Could you check a few things on this model? Use its own coordinates, in mm. A direction names the side the tool comes from. Give positions to 0.01 mm unless a question says otherwise; leave off trailing zeros. Write each loop counter-clockwise with the first axis right and the second up, starting at its lowest first coordinate (ties: lowest second). Pieces come first, ordered by that corner, then holes. Notation, with made-up numbers: (49.25, -27) - (61.25, -27) arc R26 ccw to (61.25, 12) - close; hole circle Ø2 at (39.25, 51.5). An arc over 180 degrees is marked (long way). Write item = value, one per line.
from build123d import *

# Parameters (mm, degrees)
SKETCH1_R                       = 2.5
BOSS_EXTRUDE1_DEPTH             = 25
SKETCH9_W                       = 45.48
SKETCH9_H                       = 45
BOSS_EXTRUDE4_DEPTH             = 15
CUT_EXTRUDE2_START              = -2.5
CUT_EXTRUDE2_DEPTH              = 19.5
SKETCH15_R                      = 2.5
BOSS_EXTRUDE5_DEPTH             = 25
CHAMFER1_SIZE                   = 10
CUT_EXTRUDE3_REACH              = 47.48
SKETCH16_W                      = 40
SKETCH16_H                      = 19.5
SKETCH17_W                      = 15.08
SKETCH17_H                      = 6
BOSS_EXTRUDE6_DEPTH             = 22
CBORE_FOR_M5_SBHCS1_D           = 5.5
CBORE_FOR_M5_SBHCS1_CBORE_D     = 10.5
CBORE_FOR_M5_SBHCS1_CBORE_DEPTH = 9.75
CHAMFER2_SIZE                   = 0.5


with BuildPart() as part:
    # Sketch1 → Boss-Extrude1 (new body)
    with BuildSketch(Plane(origin=(0, 0, 0), x_dir=(1, 0, 0), z_dir=(0, 1, 0))):
        Polygon((20.24, -10), (25.24, -10), (25.24, 10), (20.24, 10), (-20.24, 10), (-20.24, -10), align=None)
        Circle(SKETCH1_R, mode=Mode.SUBTRACT)
    extrude(amount=BOSS_EXTRUDE1_DEPTH)

    # Sketch9 → Boss-Extrude4 (add)
    with BuildSketch(Plane.XY.offset(10)):
        with Locations((2.5, 2.5)):
            Rectangle(SKETCH9_W, SKETCH9_H)
    extrude(amount=BOSS_EXTRUDE4_DEPTH)

    # Sketch10 → Cut-Extrude2 (cut)
    with BuildSketch(Plane(origin=(0, 25, 0), x_dir=(1, 0, 0), z_dir=(0, 1, 0)).offset(CUT_EXTRUDE2_START)):
        with BuildLine():
            Line((10.16, 0), (10.16, 10))
            Line((10.16, 10), (-10.16, 10))
            Line((-10.16, 10), (-10.16, 0))
            ThreePointArc((-10.16, 0), (0, -10.16), (10.16, 0))
        make_face()
    extrude(amount=-CUT_EXTRUDE2_DEPTH, mode=Mode.SUBTRACT)

    # Sketch15 → Boss-Extrude5 (add)
    with BuildSketch(Plane(origin=(0, 25, 0), x_dir=(1, 0, 0), z_dir=(0, 1, 0))):
        with BuildLine():
            Line((25.24, 10), (25.24, 12.732395665))
            ThreePointArc((25.24, 12.732395665), (12.732395665, 25.24), (0.224791329, 12.732395665))
            Line((0.224791329, 12.732395665), (0.224791329, 10))
            Line((0.224791329, 10), (25.24, 10))
        make_face()
        with Locations((12.732395665, 12.732395665)):
            Circle(SKETCH15_R, mode=Mode.SUBTRACT)
    extrude(amount=-BOSS_EXTRUDE5_DEPTH)

    # Chamfer1
    chamfer1_edges = [part.edges().sort_by_distance(p)[0] for p in [
        (2.5, 25, 25),
    ]]
    chamfer(chamfer1_edges, length=CHAMFER1_SIZE)

    # Sketch16 → Cut-Extrude3 (cut, up to next)
    with BuildSketch(Plane(origin=(25.24, 0, 0), x_dir=(0, 0, -1), z_dir=(1, 0, 0)), mode=Mode.PRIVATE) as cut_extrude3_sk1:
        with Locations((9.84, 12.75)):
            Rectangle(SKETCH16_W, SKETCH16_H)
    cut_extrude3_tool1 = extrude(cut_extrude3_sk1.sketch, amount=-CUT_EXTRUDE3_REACH, mode=Mode.PRIVATE) & part.part
    add(cut_extrude3_tool1.solids().sort_by_distance((25.24, 12.75, -9.84))[0], mode=Mode.SUBTRACT)

    # Sketch17 → Boss-Extrude6 (add)
    with BuildSketch(Plane(origin=(0, 25, 0), x_dir=(1, 0, 0), z_dir=(0, 1, 0))):
        with Locations((17.7, 0)):
            Rectangle(SKETCH17_W, SKETCH17_H)
    extrude(amount=-BOSS_EXTRUDE6_DEPTH)

    # CBORE for M5 SBHCS1 (through all)
    with Locations(Plane.XY.offset(25)):
        with Locations((-13.24, -10), (18.24, -10)):
            CounterBoreHole(CBORE_FOR_M5_SBHCS1_D / 2, CBORE_FOR_M5_SBHCS1_CBORE_D / 2, CBORE_FOR_M5_SBHCS1_CBORE_DEPTH)

    # Chamfer2
    chamfer2_edges = [part.edges().sort_by_distance(p)[0] for p in [
        (-20.24, 25, 2.5),
        (-20.24, -20, 17.5),
        (25.24, -20, 17.5),
        (2.5, -20, 25),
        (25.24, -2.5, 25),
        (-10.007604335, 25, -10),
        (12.732395665, 25, -25.24),
        (0.224791329, 25, -11.366197832),
        (-20.24, -2.5, 25),
        (-20.24, 20, 20),
        (25.24, 25, 1.133802168),
        (25.24, 20, 20),
    ]]
    chamfer(chamfer2_edges, length=CHAMFER2_SIZE)


solid = part.part
1. Which directions (+Z, -Z, +X, -X, +Y, -Y) give clear straight access to the entire face, cutting with the end or side of a thin tool? Please do faces 4 (the face through (18, 13, 3)), 5 (the face through (-11, -12, 15.25)), 6 (the face through (-10.16, 13, -5)), 7 (the face through (25.24, 2.8, 10.3)), 8 (the face through (-15.78, -11.05, 12.59)).
Filled sheet:
face_4 = +X
face_5 = +Z
face_6 = -Z
face_7 = +Z, -Z, +X, +Y, -Y
face_8 = +Z, -Z
2. For pin 1 (0.6 mm diameter, centred on y = 23, z = -11, fed in from -X); pin 2 (2 mm diameter, centred on x = 18.5, y = 14, fed in from -Z); pin 3 (6 mm diameter, centred on x = -10.5, y = 12.5, fed in from -Z), each with a flat end and sliding along its axis, tell me the tip position at first contact or that it passes through.
Filled sheet:
pin_1 = 0.22
pin_2 = -3
pin_3 = -10
3. If we section it at C-C, the plane z = -7.5: Please give me the cut outline in (x, y).
Filled sheet:
outline = (-20.24, 0) - (25.24, 0) - (25.24, 3) - (-10.16, 3) - (-10.16, 22.5) - (25.24, 22.5) - (25.24, 24.5) - (24.74, 25) - (-19.74, 25) - (-20.24, 24.5) - close
4. If we section it at B-B, the plane y = -10: Please give me the cut outline in (x, z).
Filled sheet:
outline = (-20.24, 10) - (-15.99, 10) - (-15.99, 15.25) - (-18.49, 15.25) - (-18.49, 25) - (-19.74, 25) - (-20.24, 24.5) - close; (-10.49, 10) - (15.49, 10) - (15.49, 15.25) - (12.99, 15.25) - (12.99, 25) - (-7.99, 25) - (-7.99, 15.25) - (-10.49, 15.25) - close; (20.99, 10) - (25.24, 10) - (25.24, 24.5) - (24.74, 25) - (23.49, 25) - (23.49, 15.25) - (20.99, 15.25) - close
5. If we section it at D-D, the plane y = 12: Please give me the cut outline in (x, z).
Filled sheet:
outline = (-20.24, -10) - (-10.16, -10) - (-10.16, 0) arc R10.16 cw to (0, 10.16) - (25.24, 10.16) - (25.24, 24.5) - (24.74, 25) - (-19.74, 25) - (-20.24, 24.5) - close; (10.16, -3) - (25.24, -3) - (25.24, 3) - (10.16, 3) - close
6. Thinking about a two-plate mould opening in Y: for faces 1 (the face through (-19.993, 19.751, 19.891)), 2 (the face through (0.225, 2, -11)), 3 (the face through (-7.263, 12.886, 7.105)), which applies, pulls with the +Y half, pulls with the -Y half, needs draft (parallel to the pull), parting line crosses it, or undercut?
Filled sheet:
face_1 = pulls with the +Y half
face_2 = needs draft
face_3 = undercut
7. I need wall thicknesses on line 1 (X direction, y = 1, z = 0); line 2 (Z direction, x = 0, y = 2.05); line 3 (Y direction, x = -13, z = 13). Which ranges of each line are inside material? Lowest first, please.
Filled sheet:
line_1 = -20.24 to -2.5, 2.5 to 25.24
line_2 = -10 to -2.5, 2.5 to 25
line_3 = -20 to -12.74, -7.26 to 25
8. If we section it at A-A, the plane x = -13.24: Please give me the cut outline in (y, z), and give its area (4 significant figures).
Filled sheet:
outline = (-20, 10) - (-12.75, 10) - (-12.75, 15.25) - (-15.25, 15.25) - (-15.25, 25) - (-19.5, 25) - (-20, 24.5) - close; (-7.25, 10) - (0, 10) - (0, -10) - (24.5, -10) - (25, -9.5) - (25, 15) - (15, 25) - (-4.75, 25) - (-4.75, 15.25) - (-7.25, 15.25) - close
area = 993.5 mm2
